Solid Edge part; units mm, degrees
sketch "Sketch1" plane through (0, 0, 0) normal (0, -1, 0) x (1, 0, 0)
  line L0 (1.5, 0) -> (3, 1.5)
  line L1 (3, 1.5) -> (3, 1.7)
  line L2 (3, 1.7) -> (0, 1.7)
  line L3 (0, 1.7) -> (0, -28.3)
  line L4 (0, -28.3) -> (1.1935, -28.3)
  line L5 (1.1935, -28.3) -> (1.5, -27.9935)
  line L6 (1.5, -27.9935) -> (1.5, -16.3)
  line L7 (1.5, -16.3) -> (1.1935, -16.3)
  line L8 (1.1935, -16.3) -> (1.1935, -16.29)
  line L9 (1.1935, -16.29) -> (1.5, -16.29)
  line L10 (1.5, -16.29) -> (1.5, 0)
  dimension "D1" = 1.5
  dimension "D2" = 1.1935
revolve "RevolvedProtrusion1" add sketch "Sketch1" angle 360 about axis through (0, 0, 54) along (0, 0, -1)
sketch "Sketch2" plane through (0, 0, 0) normal (0, -1, 0) x (1, 0, 0)
  arc A0 (-1, 0.5) -> (0, 0) centre (0, 1.25) ccw
  line L0 (0, 0.5) -> (0, 0)
  line L1 (-1, 0.5) -> (0, 0.5)
revolve "RevolvedCutout1" cut sketch "Sketch2" angle 360 about axis through (0, 0, 54) along (0, 0, -1)
sketch "Sketch3" plane through (0, 0, 1.7) normal (0, 0, 1) x (0, -1, 0)
  line L0 (-1.1547, 0) -> (-0.5774, 1)
  line L1 (-0.5774, 1) -> (0.5774, 1)
  line L2 (0.5774, 1) -> (1.1547, 0)
  line L3 (1.1547, 0) -> (0.5774, -1)
  line L4 (0.5774, -1) -> (-0.5774, -1)
  line L5 (-0.5774, -1) -> (-1.1547, 0)
extrude "Cutout1" cut sketch "Sketch3" against normal blind 1.2
cosmetic_thread "Thread1"
sketch "Sketch4" plane through (0, 0, 0) normal (1, 0, 0) x (0, 1, 0)
  line L0 (-1.15, 1.7) -> (0, 1.036)
revolve "RevolvedCutout2" cut sketch "Sketch4" angle 360 about axis through (0, 0, -57) along (0, 0, 1) material side at (0, -0.55, 1.4113)
fillet "Round1" radius 0.1 1 edges at (-1.5, 0, 0)
sketch "Sketch5" plane through (0, 0, 0) normal (1, 0, 0) x (0, 1, 0)
  line L0 (-2.6438, -25.3) -> (2.8741, -25.3)
extrude "Extrusionsausschnitt_2" cut sketch "Sketch5" along normal mid plane 108.2201 material side at (0, 0.1151, -25.35)
chamfer "Fase_1" distance 0.31 angle 45 1 edges at (-1.5, 0, -25.3)
properties material "Stahl"
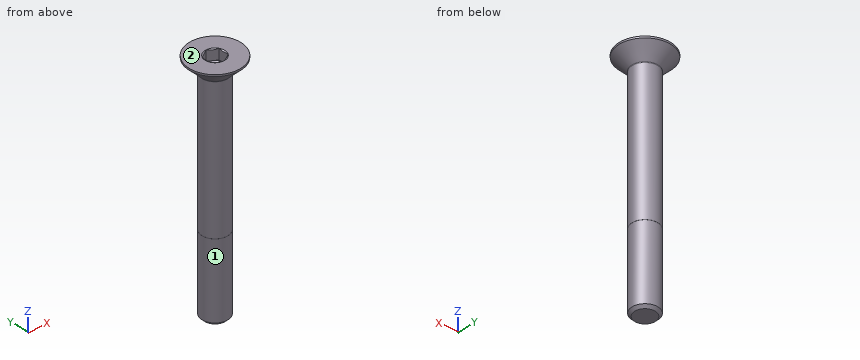
Design review of the part built by this model. Coordinates are the model's own, in mm. Face numbers are marked on the shaded views. A direction names the side the tool comes from. Give positions to 0.01 mm unless a question says otherwise; leave off trailing zeros. Write each loop counter-clockwise with the first axis right and the second up, starting at its lowest first coordinate (ties: lowest second). Pieces come first, ordered by that corner, then holes.
(1) Wall thickness on line 1 along Z through (x, y) = (2, 1.5); line 2 along X through (y, z) = (0, -10.75); line 3 along Z through (x, y) = (0.25, 0): over which ranges is each line inside the solid? List them lowest first.
Checked values:
line 1: z = 1 to 1.7
line 2: x = -1.5 to 1.5
line 3: z = -25.3 to 0.03
(2) Add section A-A (z = -4). Give the boundary of the cut face in (x, y).
Checked values:
outline: circle Ø3 at (0, 0)
(3) Tool access review of the marked faces 1 and 2: name each direction out of +Z, -Z, +X, -X, +Y, -Y from which nothing blocks a thin tool from reaching the whole face with its end or side.
Checked values:
face 1: -Z
face 2: +Z, +X, -X, +Y, -Y
(4) Clearance check with flat-ended pins moving along their axes: pin 1 Ø1.5 at (y, z) = (0.5, -15) entering from -X; pin 2 Ø1.5 at (x, z) = (-1.5, -13.5) entering from +Y. State where each tip first meets the part, or that it passes through.
Checked values:
pin 1: stops at x = -1.5
pin 2: stops at y = 1.3
